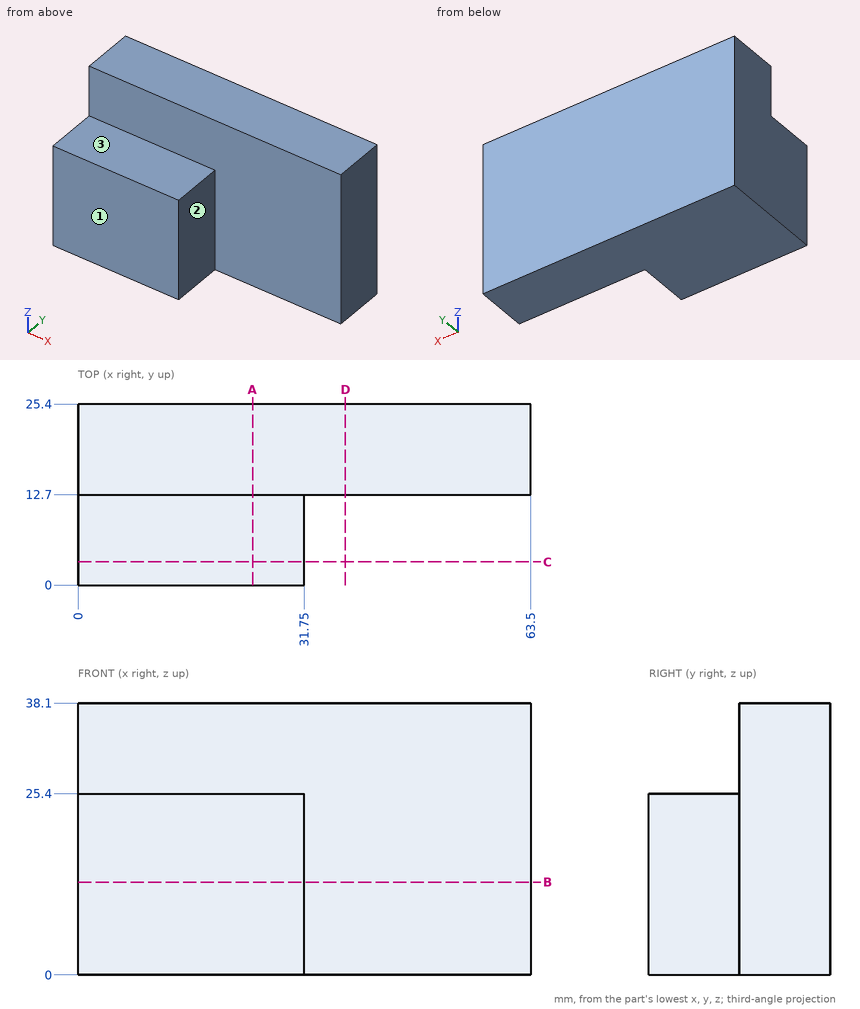
Geometry: see drawing. Coordinates: mm, zero at the bounding-box minimum. A direction names the side the tool comes from. Round coordinates to 2 decimals unless told otherwise and drop trailing zeros. Write each loop counter-clockwise with the first axis right and the second up, starting at its lowest first coordinate (ties: lowest second). Pieces come first, ordered by that corner, then holes. Notation, with made-up numbers: M 22,71 L 53,71 A33 ccw 53,103 Z; hole C -17,73 d9. An arc over 180 degrees is marked long. Answer as a JSON object with one key per item and string values. Group by question number.
(1) Reachability of the marked faces 1, 2 and 3 from +Z, -Z, +X, -X, +Y, -Y: full face, straight path, thin tool, end or side. Return the list, or none.
(2) Section query C-C on y = 3.25. Output: boundary loops of the cut face in (x, z), then the cut area to 3 significant figures.
(3) Section query B-B on z = 13. Output: boundary loops of the cut face in (x, y), then the cut area to 3 significant figures.
(4) First-contact query: pin 1 (12 mm diameter, centred on x = 38.5, z = 29, fed in from -Y); pin 2 (1 mm diameter, centred on y = 5, z = 11.5, fed in from +X); pin 3 (4 mm diameter, centred on x = 19, y = 9, fed in from +Z). Flat tips, straight axial feed; report the tip coordinate or a pass-through.
(5) Section query D-D on x = 37.5. Output: boundary loops of the cut face in (y, z), then the cut area to 3 significant figures.
(6) Ray query, line 1 (Y direction, x = 6.5, z = 37.5); line 2 (X direction, y = 3, z = 4.5); line 3 (Z direction, x = 9, y = 6.5). Return the intervals inside material, ascending. Write a range as [from, to].
(7) Section query A-A on x = 24.5. Output: boundary loops of the cut face in (y, z).
Computed values:
{
 "1": {"face 1": "+Z, -Z, +X, -X, -Y", "face 2": "+Z, -Z, +X, -Y", "face 3": "+Z, +X, -X, -Y"},
 "2": {"outline": "M 0,0 L 31.75,0 L 31.75,25.4 L 0,25.4 Z", "area": "806 mm^2"},
 "3": {"outline": "M 0,0 L 31.75,0 L 31.75,12.7 L 63.5,12.7 L 63.5,25.4 L 0,25.4 Z", "area": "1,210 mm^2"},
 "4": {"pin 1": "y = 12.7", "pin 2": "x = 31.75", "pin 3": "z = 25.4"},
 "5": {"outline": "M 12.7,0 L 25.4,0 L 25.4,38.1 L 12.7,38.1 Z", "area": "484 mm^2"},
 "6": {"line 1": "[12.7, 25.4]", "line 2": "[0, 31.75]", "line 3": "[0, 25.4]"},
 "7": {"outline": "M 0,0 L 25.4,0 L 25.4,38.1 L 12.7,38.1 L 12.7,25.4 L 0,25.4 Z"}
}
